Check sheet for the drawn part. Datum: minimum x, y, z corner. Units: mm. A direction names the side the tool comes from. Give positions to 0.01 mm unless a question says otherwise; leave off trailing zeros. Write each loop counter-clockwise with the first axis right and the second up, starting at its lowest first coordinate (ties: lowest second). Pieces come first, ordered by that corner, then holes. Notation, with made-up numbers: (66, 78.5) -> (72, 78.5) arc R12 ccw to (72, 82.5) -> close; hole circle Ø11 at (-29.75, 63.5). An arc over 180 degrees is marked (long way). Write item = value, one per line. Start each with the question number.
1. Cross-section at D-D, the plane y = 11.75. Record the cut outline in (x, z).
2. Thickness scan on line 1 along X through (y, z) = (11.5, 13.75) (1 decimal); line 2 along Y through (x, z) = (26.25, 19.5); line 3 along Z through (x, y) = (13.5, 4.25) (1 decimal). Record the ranges inside material, lowest first.
3. Cross-section at A-A, the plane z = 26. Record the cut outline in (x, y) (1 decimal), plus the area to 3 significant figures.
4. Cross-section at C-C, the plane y = 2. Record the cut outline in (x, z).
5. Cross-section at B-B, the plane x = 24.5. Record the cut outline in (y, z).
6. Mould release check, pull along Z, two halves, no side actions. Record for the marked faces 4, 5 and 6: pulls with the +Z half, pulls with the -Z half, needs draft (parallel to the pull), parting line crosses it, or undercut.
7. Set-up check for the marked faces 1, 2 and 3: record each of +Z, -Z, +X, -X, +Y, -Y from which the full face is reachable in a straight line by a thin tool's end or side.
8. Depth check by flat-ended pin: P1, Ø8, axis at x = 8, z = 6, coming from the +Y side; P2, Ø3, axis at x = 21.5, y = 8.5, coming from the -Z side; P3, Ø3, axis at x = 3.85, z = 8.06, coming from the -Y side; P4, Ø3.5, axis at x = 23.8, z = 8.06, coming from the +Y side. Enter the tip coordinate at first touch or a pass-through.
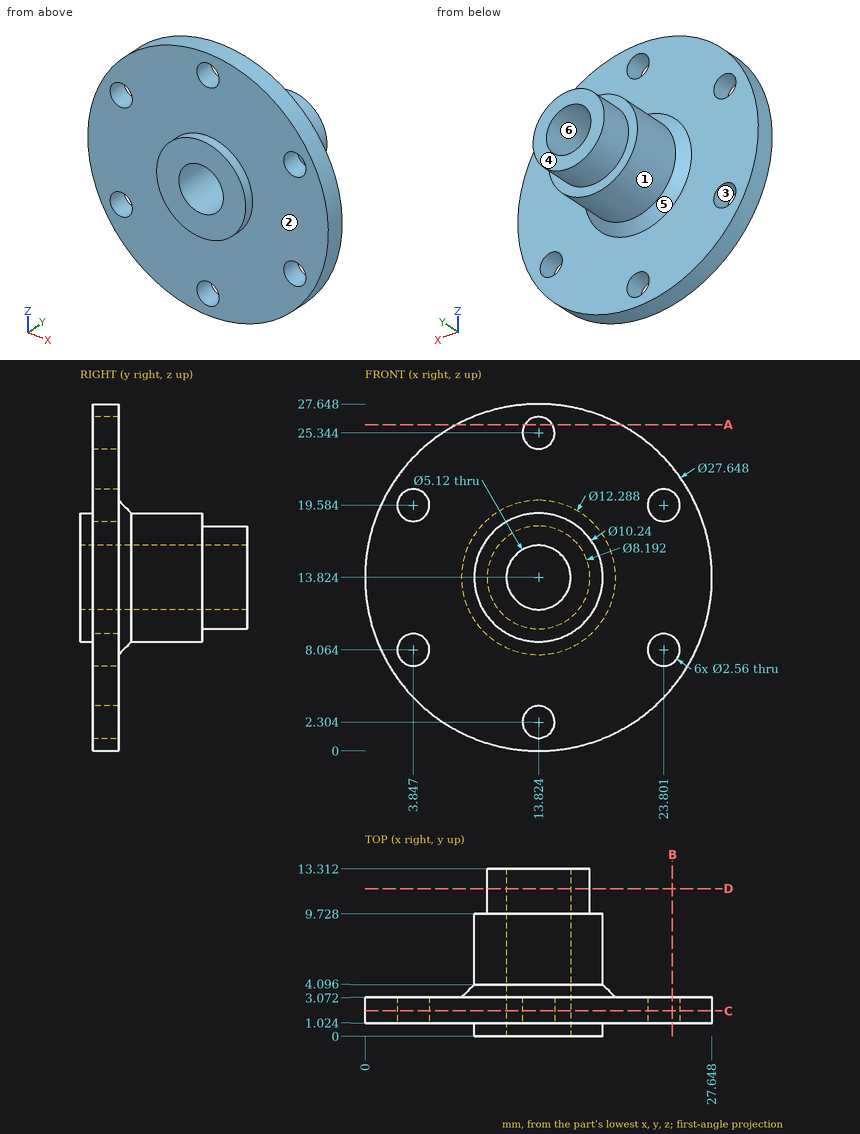
Answers:
q1.outline = circle Ø8.19 at (13.82, 13.82); hole circle Ø5.12 at (13.82, 13.82)
q2.line_1 = 9.7 to 11.3, 16.4 to 17.9
q2.line_2 = 1.02 to 3.07
q2.line_3 = 8.7 to 11.3, 16.4 to 18.9
q3.outline = (7.3, 1) -> (12.7, 1) -> (12.7, 3.1) -> (7.3, 3.1) -> close; (14.9, 1) -> (20.4, 1) -> (20.4, 3.1) -> (14.9, 3.1) -> close
q3.area = 22.3 mm^2
q4.outline = circle Ø27.65 at (13.82, 13.82); hole circle Ø2.56 at (3.85, 8.06); hole circle Ø2.56 at (3.85, 19.58); hole circle Ø5.12 at (13.82, 13.82); hole circle Ø2.56 at (13.82, 2.3); hole circle Ø2.56 at (13.82, 25.34); hole circle Ø2.56 at (23.8, 8.06); hole circle Ø2.56 at (23.8, 19.58)
q5.outline = (1.02, 5.04) -> (3.07, 5.04) -> (3.07, 6.99) -> (1.02, 6.99) -> close; (1.02, 9.14) -> (3.07, 9.14) -> (3.07, 18.51) -> (1.02, 18.51) -> close; (1.02, 20.66) -> (3.07, 20.66) -> (3.07, 22.61) -> (1.02, 22.61) -> close
q6.face_4 = needs draft
q6.face_5 = parting line crosses it
q6.face_6 = undercut
q7.face_1 = +Y
q7.face_2 = -Y
q7.face_3 = +Y, -Y
q8.P1 = 3.46
q8.P2 = through
q8.P3 = 1.02
q8.P4 = 3.07
